Part model, mm, in its own coordinate system. A direction names the side the tool comes from. Coordinates: 2 decimals unless noted, no trailing zeros. Write each loop counter-clockwise with the first axis right and the second up, starting at its lowest first coordinate (ties: lowest second). Pieces come first, ordered by that corner, then holes. Notation, with made-up numbers: M 86,-28 L 103,-28 A13 ccw 103,-10 Z; hole C 66,50 d11. An arc over 180 degrees is marked long. Use a Markdown table: item, result. Add a question column.
Q1. Slice it at B-B on y = -4. Write the cut outline in (x, z) (3 decimals), then the cut area to 3 significant figures.
Q2. Slice it at A-A on x = -18. Write the cut outline in (y, z) (3 decimals).
Q3. Mould opens along X. For faces 5 (the cylindrical face through (35.454, 11.896, 0.93)), 6 (the cylindrical face through (-45.265, -6.971, 0.567)), 7 (the cylindrical face through (48.636, -0.339, 2.449)) say: released by +X, released by -X, zero draft, split by the parting line, or undercut.
Q4. Tool access for faces 1 (the cylindrical face through (47.137, -0.306, 3.119)), 2 (the flat face through (-37, 0, 1.15)), 3 (the cylindrical face through (-45.167, 7.138, 0.567)), 4 (the flat face through (-35, 0, 2)): list every direction of +Z, -Z, +X, -X, +Y, -Y with a clear straight run to the whole face (end or side of a thin tool).
Q5. Pin check, flat tips, straight feed: pin 1 Ø0.6 at (y, z) = (-12.5, 1) entering from +X; pin 2 Ø0.6 at (x, z) = (-45.5, 0.5) entering from +Y; pin 3 Ø5.5 at (x, y) = (-39.5, -5.5) entering from -Z. Stop position of each tip, or through.
Q6. Wall check: L1, parallel to Y at x = 14.5, z = 2.95; L2, parallel to X at y = 0.5, z = 1.25; L3, parallel to X at y = 0.5, z = 2.9. Give the ranges that are in metal, low to high. Write a range as from..to.
from build123d import *

# Parameters (mm, degrees)
PAD_DEPTH       = 1.15
SKETCH001_W     = 1
SKETCH001_H     = 0.51
SKETCH001_W_2   = 0.51
SKETCH001_H_2   = 1
POCKET_DEPTH    = 1.15
PAD001_DEPTH    = 2.635
SKETCH003_R     = 2.375
PAD002_DEPTH    = 2.635
POCKET001_DEPTH = 1.35


with BuildPart() as part:
    # Sketch → Pad (new body)
    with BuildSketch(Plane.XY):
        with BuildLine():
            Line((-33.24, 13.9), (33.24, 13.9))
            ThreePointArc((33.24, -13.9), (47.14, 0), (33.24, 13.9))
            Line((-33.24, -13.9), (33.24, -13.9))
            ThreePointArc((-33.24, 13.9), (-47.14, 0), (-33.24, -13.9))
        make_face()
        with BuildLine():
            Line((-33.24, 12.1), (33.24, 12.1))
            ThreePointArc((33.24, -12.1), (45.34, 0), (33.24, 12.1))
            Line((-33.24, -12.1), (33.24, -12.1))
            ThreePointArc((-33.24, 12.1), (-45.34, 0), (-33.24, -12.1))
        make_face(mode=Mode.SUBTRACT)
    extrude(amount=PAD_DEPTH)

    # Sketch001 (on Face9 of Pad) → Pocket (cut)
    with BuildSketch(Plane(origin=(0, 0, 0), x_dir=(1, 0, 0), z_dir=(0, 0, -1))):
        with Locations((0, 12.355)):
            Rectangle(SKETCH001_W, SKETCH001_H)
        with Locations((0, 13.645)):
            Rectangle(SKETCH001_W, SKETCH001_H)
        with Locations((0, -12.355)):
            Rectangle(SKETCH001_W, SKETCH001_H)
        with Locations((0, -13.645)):
            Rectangle(SKETCH001_W, SKETCH001_H)
        with Locations((45.584665, 0)):
            Rectangle(SKETCH001_W_2, SKETCH001_H_2)
        with Locations((46.885, 0)):
            Rectangle(SKETCH001_W_2, SKETCH001_H_2)
        with Locations((-45.584665, 0)):
            Rectangle(SKETCH001_W_2, SKETCH001_H_2)
        with Locations((-46.885, 0)):
            Rectangle(SKETCH001_W_2, SKETCH001_H_2)
        Polygon((39.538496, 10.331454), (38.663876, 10.816264), (38.911129, 11.26232), (39.785749, 10.777511), align=None)
        Polygon((40.416164, 11.914809), (39.541544, 12.399619), (39.294291, 11.953563), (40.168911, 11.468753), align=None)
        Polygon((38.663876, -10.816264), (39.538496, -10.331454), (39.785749, -10.777511), (38.911129, -11.26232), align=None)
        Polygon((39.541544, -12.399619), (40.416164, -11.914809), (40.168911, -11.468753), (39.294291, -11.953563), align=None)
        Polygon((-39.538496, 10.331454), (-38.663876, 10.816264), (-38.911129, 11.26232), (-39.785749, 10.777511), align=None)
        Polygon((-40.416164, 11.914809), (-39.541544, 12.399619), (-39.294291, 11.953563), (-40.168911, 11.468753), align=None)
        Polygon((-39.541544, -12.399619), (-40.416164, -11.914809), (-40.168911, -11.468753), (-39.294291, -11.953563), align=None)
        Polygon((-38.663876, -10.816264), (-39.538496, -10.331454), (-39.785749, -10.777511), (-38.911129, -11.26232), align=None)
    extrude(amount=-POCKET_DEPTH, mode=Mode.SUBTRACT)

    # Sketch002 (on Face4 of Pocket) → Pad001 (join)
    with BuildSketch(Plane.XY.offset(1.15)):
        with BuildLine():
            Line((-33.24, 15.4), (33.24, 15.4))
            ThreePointArc((33.24, -15.4), (48.64, 0), (33.24, 15.4))
            Line((-33.24, -15.4), (33.24, -15.4))
            ThreePointArc((-33.24, 15.4), (-48.64, 0), (-33.24, -15.4))
        make_face()
        with BuildLine():
            ThreePointArc((-33.24, 12.1), (-45.34, 0), (-33.24, -12.1))
            Line((-33.24, -12.1), (33.24, -12.1))
            ThreePointArc((33.24, -12.1), (45.34, 0), (33.24, 12.1))
            Line((33.24, 12.1), (-33.24, 12.1))
        make_face(mode=Mode.SUBTRACT)
    extrude(amount=PAD001_DEPTH)

    # Sketch003 (on Face4 of Pocket) → Pad002 (join)
    with BuildSketch(Plane.XY.offset(1.15)):
        with BuildLine():
            ThreePointArc((-35, 11.971316), (-45.34, 0), (-35, -11.971316))
            Line((-35, 11.971316), (-35, -11.971316))
        make_face()
        with Locations((-40.25, 0)):
            Circle(SKETCH003_R, mode=Mode.SUBTRACT)
        with BuildLine():
            Line((35, -11.971316), (35, 11.971316))
            ThreePointArc((35, -11.971316), (45.34, 0), (35, 11.971316))
        make_face()
        with Locations((40.25, 0)):
            Circle(SKETCH003_R, mode=Mode.SUBTRACT)
    extrude(amount=PAD002_DEPTH)

    # Sketch004 (on Face95 of Pad002) → Pocket001 (cut)
    with BuildSketch(Plane.XY.offset(3.785)):
        with BuildLine():
            ThreePointArc((-33.24, 13.9), (-47.14, 0), (-33.24, -13.9))
            Line((-33.24, -13.9), (33.24, -13.9))
            ThreePointArc((33.24, -13.9), (47.14, 0), (33.24, 13.9))
            Line((33.24, 13.9), (-33.24, 13.9))
        make_face()
        with BuildLine():
            ThreePointArc((-33.24, 12.1), (-45.34, 0), (-33.24, -12.1))
            Line((-33.24, -12.1), (33.24, -12.1))
            ThreePointArc((33.24, -12.1), (45.34, 0), (33.24, 12.1))
            Line((-33.24, 12.1), (33.24, 12.1))
        make_face(mode=Mode.SUBTRACT)
    extrude(amount=-POCKET001_DEPTH, mode=Mode.SUBTRACT)


solid = part.part
Recorded:
| question | item | result |
|---|---|---|
| 1 | outline | M -48.111,1.15 L -46.552,1.15 L -46.552,0 L -44.66,0 L -44.66,1.15 L -35,1.15 L -35,3.785 L -44.66,3.785 L -44.66,2.435 L -46.552,2.435 L -46.552,3.785 L -48.111,3.785 Z; M 35,1.15 L 44.66,1.15 L 44.66,0 L 46.552,0 L 46.552,1.15 L 48.111,1.15 L 48.111,3.785 L 46.552,3.785 L 46.552,2.435 L 44.66,2.435 L 44.66,3.785 L 35,3.785 Z |
| 1 | area | 68.3 mm² |
| 2 | outline | M -15.4,1.15 L -13.9,1.15 L -13.9,0 L -12.1,0 L -12.1,2.435 L -13.9,2.435 L -13.9,3.785 L -15.4,3.785 Z; M 12.1,0 L 13.9,0 L 13.9,1.15 L 15.4,1.15 L 15.4,3.785 L 13.9,3.785 L 13.9,2.435 L 12.1,2.435 Z |
| 3 | face 5 | undercut |
| 3 | face 6 | released by -X |
| 3 | face 7 | released by +X |
| 4 | face 1 | +Z |
| 4 | face 2 | -Z |
| 4 | face 3 | -Z, -X, +Y |
| 4 | face 4 | +Z, -Z |
| 5 | pin 1 | x = 42.59 |
| 5 | pin 2 | y = 7.08 |
| 5 | pin 3 | z = 1.15 |
| 6 | L1 | -15.4..-13.9, 13.9..15.4 |
| 6 | L2 | -48.63..-42.57, -37.93..-35, 35..37.93, 42.57..48.63 |
| 6 | L3 | -48.63..-47.13, -45.33..-42.57, -37.93..-35, 35..37.93, 42.57..45.33, 47.13..48.63 |
